```python
from build123d import *

# Parameters (mm, degrees)
F1_DEPTH      = 42
F2_T          = -3.5
F3_W          = 40
F3_H          = 75
F4_DEPTH      = 4
F6_DEPTH      = 5
F8_W          = 9
F8_H          = 9
F9_DEPTH      = 20.5
F10_DEPTH     = 32
F12_R         = 6
F13_DEPTH     = 25
F15_W         = 8.3580343053
F15_H         = 30.4632759653
F15_W_2       = 12.1421813965
F15_H_2       = 30.5070821196
F16_DEPTH     = 6
F17_T1_DEPTH  = 169.3882617949
F17_T3_DEPTH  = 92.6602540378
F17_T5_DEPTH  = 46.118363099
F17_T7_DEPTH  = 35
F18_D         = 2.5
F18_DEPTH     = 18
F18_TIP       = 0.7510757738
F19_T1_DEPTH  = 80
F19_T6_DEPTH  = 2
F19_T12_DEPTH = 2
F20_D         = 2.5
F20_DEPTH     = 18
F20_TIP       = 0.7510757738


# Not quite as in the source:
# - a fillet or chamfer that OpenCascade refuses, or shapes differently, is made with other operations: its cross-section is extruded or revolved along the edge and cut away or added
# - a feature names something its author has since deleted; it is built from what else it names


with BuildPart() as f1:
    # F0 (on Front) → F1 (new body, symmetric)
    with BuildSketch(Plane.XZ):
        Polygon((-66.6393345791, 36.118363099), (-66.6393345791, 0), (93.3606654209, 0), (93.3606654209, 25), (-65.6393345791, 36.118363099), align=None)
    extrude(amount=F1_DEPTH, both=True)

    # F2
    f2_openings = [f1.faces().sort_by_distance(p)[0] for p in [
        (13.360665, 0, 0),
    ]]
    offset(amount=F2_T, openings=f2_openings)

    # F3 (on face) → F4 (cut)
    with BuildSketch(Plane(origin=(2.1939535511, 0, 31.3749975164), x_dir=(0.9975640503, 0, -0.0697564737), z_dir=(0.0697564737, 0, 0.9975640503))):
        with Locations((-20.9989301063, 0)):
            Rectangle(F3_W, F3_H)
    extrude(amount=-F4_DEPTH, mode=Mode.SUBTRACT)

    # F3 (on face) → F6 (cut)
    with BuildSketch(Plane(origin=(2.1939535511, 0, 31.3749975164), x_dir=(0.9975640503, 0, -0.0697564737), z_dir=(0.0697564737, 0, 0.9975640503))):
        with BuildLine():
            Line((14.9393316886, 27.279802623), (14.9393316886, 22.720197377))
            ThreePointArc((14.9393316886, 22.720197377), (19.3893316886, 20), (23.8393316886, 22.720197377))
            Line((23.8393316886, 22.720197377), (23.8393316886, 27.279802623))
            ThreePointArc((23.8393316886, 27.279802623), (19.3893316886, 30), (14.9393316886, 27.279802623))
        make_face()
        with BuildLine():
            Line((20.0393316886, -34.0238362551), (20.0393316886, -33.0238362551))
            ThreePointArc((20.0393316886, -33.0238362551), (19.3893316886, -16.9498789917), (18.7393316886, -33.0238362551))
            Line((18.7393316886, -33.0238362551), (18.7393316886, -34.0238362551))
            Line((18.7393316886, -34.0238362551), (20.0393316886, -34.0238362551))
        make_face()
    extrude(amount=-F6_DEPTH, mode=Mode.SUBTRACT)

    # F8 (on offset) → F9 (join)
    with BuildSketch(Plane(origin=(0, 0, 2.5), x_dir=(1, 0, 0), z_dir=(0, 0, -1))):
        with Locations((81.6606654209, 34)):
            Rectangle(F8_W, F8_H)
        with Locations((81.6606654209, -34)):
            Rectangle(F8_W, F8_H)
    extrude(amount=-F9_DEPTH)

    # F8 (on offset) → F10 (join)
    with BuildSketch(Plane(origin=(0, 0, 2.5), x_dir=(1, 0, 0), z_dir=(0, 0, -1))):
        with Locations((-58.6393345791, -34)):
            Rectangle(F8_W, F8_H)
        with Locations((-58.6393345791, 34)):
            Rectangle(F8_W, F8_H)
    extrude(amount=-F10_DEPTH)

    # F12 (on offset) → F13 (cut)
    with BuildSketch(Plane(origin=(-66.6393345791, 0, 0), x_dir=(0, -1, 0), z_dir=(-1, 0, 0))):
        with Locations((-22, 23)):
            Circle(F12_R)
        with Locations((22, 23)):
            Circle(F12_R)
    extrude(amount=-F13_DEPTH, mode=Mode.SUBTRACT)

    # F15 (on offset) → F16 (join)
    with BuildSketch(Plane(origin=(1.949805893, 0, 27.8835233405), x_dir=(0.9975640503, 0, -0.0697564737), z_dir=(-0.0697564737, 0, -0.9975640503))):
        with Locations((5.292899441, 1.1196539272)):
            Rectangle(F15_W, F15_H)
        with Locations((44.2803874612, 1.1346279643)):
            Rectangle(F15_W_2, F15_H_2)
    extrude(amount=F16_DEPTH)

    # F17: fillet of radius 2 on 7 edges, made by hand

    # F17_s2 → F17_t1 (cut)
    with BuildSketch(Plane(origin=(96.1545321211, 0, -6.7237798852), x_dir=(0, 1, 0), z_dir=(-0.9975640503, 0, 0.0697564737))):
        with BuildLine():
            ThreePointArc((40, -31.4516120627), (41.4142135624, -30.865825625), (42, -29.4516120627))
            Line((42, -29.4516120627), (42, -31.4516120627))
            Line((42, -31.4516120627), (40, -31.4516120627))
        make_face()
        with BuildLine():
            ThreePointArc((-40, -31.4516120627), (-41.4142135624, -30.865825625), (-42, -29.4516120627))
            Line((-42, -29.4516120627), (-42, -31.4516120627))
            Line((-42, -31.4516120627), (-40, -31.4516120627))
        make_face()
    extrude(amount=F17_T1_DEPTH, mode=Mode.SUBTRACT)

    # F17_s4 → F17_t3 (cut)
    with BuildSketch(Plane.XZ.offset(-46.3301270189)):
        with BuildLine():
            ThreePointArc((-65.6393345791, 36.118363099), (-66.3713853867, 35.3863122914), (-66.6393345791, 34.3863122914))
            Line((-66.6393345791, 34.3863122914), (-66.6393345791, 36.118363099))
            Line((-66.6393345791, 36.118363099), (-65.6393345791, 36.118363099))
        make_face()
    extrude(amount=F17_T3_DEPTH, mode=Mode.SUBTRACT)

    # F17_s6 → F17_t5 (cut)
    with BuildSketch(Plane.XY.offset(-5)):
        with BuildLine():
            ThreePointArc((-64.6393345791, 42), (-66.0535481415, 41.4142135624), (-66.6393345791, 40))
            Line((-66.6393345791, 40), (-66.6393345791, 42))
            Line((-66.6393345791, 42), (-64.6393345791, 42))
        make_face()
        with BuildLine():
            ThreePointArc((-64.6393345791, -42), (-66.0535481415, -41.4142135624), (-66.6393345791, -40))
            Line((-66.6393345791, -40), (-66.6393345791, -42))
            Line((-66.6393345791, -42), (-64.6393345791, -42))
        make_face()
    extrude(amount=F17_T5_DEPTH, mode=Mode.SUBTRACT)

    # F17_s8 → F17_t7 (cut)
    with BuildSketch(Plane.XY.offset(-5)):
        with BuildLine():
            ThreePointArc((91.3606654209, 42), (92.7748789833, 41.4142135624), (93.3606654209, 40))
            Line((93.3606654209, 40), (93.3606654209, 42))
            Line((93.3606654209, 42), (91.3606654209, 42))
        make_face()
        with BuildLine():
            ThreePointArc((93.3606654209, -40), (92.7748789833, -41.4142135624), (91.3606654209, -42))
            Line((91.3606654209, -42), (93.3606654209, -42))
            Line((93.3606654209, -42), (93.3606654209, -40))
        make_face()
    extrude(amount=F17_T7_DEPTH, mode=Mode.SUBTRACT)

    # F18
    with Locations(Plane(origin=(0, 0, 2.5), x_dir=(1, 0, 0), z_dir=(0, 0, -1))):
        with Locations((-58.6393345791, 34), (-58.6393345791, -34)):
            Hole(F18_D / 2, depth=F18_DEPTH)
            with Locations((0, 0, -(F18_DEPTH + F18_TIP / 2))):  # 118° drill point
                Cone(0, F18_D / 2, F18_TIP, mode=Mode.SUBTRACT)

    # F19: fillet of radius 2 on 1 edges, made by hand

    # F19_s2 → F19_t1 (cut)
    with BuildSketch(Plane.XZ.offset(-40)):
        with BuildLine():
            ThreePointArc((91.5001783684, 25.1300979282), (92.8233728241, 24.4989665478), (93.3606654209, 23.1349698277))
            Line((93.3606654209, 23.1349698277), (93.3606654209, 25))
            Line((93.3606654209, 25), (91.5001783684, 25.1300979282))
        make_face()
    extrude(amount=F19_T1_DEPTH, mode=Mode.SUBTRACT)


with BuildPart() as f19_tool4:
    # F19_s5 → F19_t6 (new body)
    with BuildSketch(Plane.XZ.offset(40)):
        Polygon((91.3606654209, 23.1349698277), (91.5001783684, 25.1300979282), (93.3606654209, 25), (93.3606654209, 23.1349698277), align=None)
    extrude(amount=F19_T6_DEPTH)

    # F19_s7 → F19_t8 (revolve, cut)
    with BuildSketch(Plane(origin=(91.3606654209, -40, 23.1349698277), x_dir=(-0.7313537016, 0, -0.6819983601), z_dir=(-0.6819983601, 0, 0.7313537016))):
        with BuildLine():
            ThreePointArc((0, -2), (2, 0), (0, 2))
            Line((0, 2), (0, -2))
        make_face()
    revolve(axis=Axis((91.3606654209, -40, 23.1349698277), (0, -1, 0)), mode=Mode.SUBTRACT)


with BuildPart() as f1_1:
    add(f1.part)

    # F19_t3: cut F19_tool4
    add(f19_tool4.part, mode=Mode.SUBTRACT)


with BuildPart() as f19_tool10:
    # F19_s11 → F19_t12 (new body)
    with BuildSketch(Plane.XZ.offset(-40)):
        Polygon((91.3606654209, 23.1349698277), (91.5001783684, 25.1300979282), (93.3606654209, 25), (93.3606654209, 23.1349698277), align=None)
    extrude(amount=-F19_T12_DEPTH)

    # F19_s13 → F19_t14 (revolve, cut)
    with BuildSketch(Plane(origin=(91.3606654209, 40, 23.1349698277), x_dir=(-0.7313537016, 0, -0.6819983601), z_dir=(0.6819983601, 0, -0.7313537016))):
        with BuildLine():
            ThreePointArc((0, -2), (2, 0), (0, 2))
            Line((0, 2), (0, -2))
        make_face()
    revolve(axis=Axis((91.3606654209, 40, 23.1349698277), (0, 1, 0)), mode=Mode.SUBTRACT)


with BuildPart() as f1_2:
    add(f1_1.part)

    # F19_t9: cut F19_tool10
    add(f19_tool10.part, mode=Mode.SUBTRACT)

    # F20
    with Locations(Plane(origin=(0, 0, 2.5), x_dir=(1, 0, 0), z_dir=(0, 0, -1))):
        with Locations((81.6606654209, 34), (81.6606654209, -34)):
            Hole(F20_D / 2, depth=F20_DEPTH)
            with Locations((0, 0, -(F20_DEPTH + F20_TIP / 2))):  # 118° drill point
                Cone(0, F20_D / 2, F20_TIP, mode=Mode.SUBTRACT)


solid = f1_2.part
```
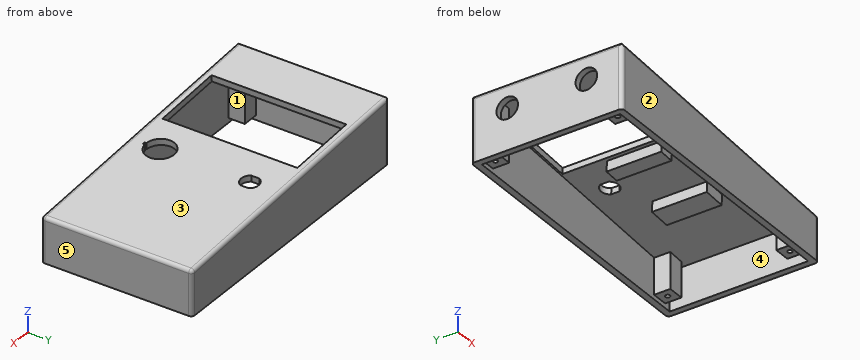
Geometry check sheet. Reference: the model listing, model coordinates, mm. Face numbers are marked on the shaded views. A direction names the side the tool comes from. Coordinates: 2 decimals unless noted, no trailing zeros. Loops run counter-clockwise (first coordinate to the right, second up) from the corner with the lowest first, then second, coordinate; pieces in that order, holes last. Notation, with made-up numbers: (-18.5, 71) - (12.5, 71) arc R32 cw to (12.5, 102) - close; hole circle Ø8 at (64.25, -8). An arc over 180 degrees is marked (long way). One line per item, written item: value. Start each with the question number.
(1) Cross-section at A-A on z = 13. Enter the section's corners in (x, y).
(2) Mould release check, pull along X, two halves, no side actions. Record for the marked faces 1, 2 and 3: released by +X, released by -X, zero draft, split by the parting line, or undercut.
(3) Cross-section at B-B on y = -18.5. Enter the section's corners in (x, z) (3 decimals).
(4) Depth check by flat-ended pin: P1, Ø2, axis at x = -58.64, y = -34, coming from the -Z side; P2, Ø4.5, axis at x = -56.5, y = 32, coming from the -Z side; P3, Ø1.5, axis at x = 54.5, y = 12.5, coming from the +Z side. Enter the tip coordinate at first touch or a pass-through.
(5) Cross-section at C-C on y = 24.5. Enter the section's corners in (x, z) (3 decimals).
(6) Tool access check on the marked faces 4 and 5. Record the directions out of +Z, -Z, +X, -X, +Y, -Y that give a thin tool (end or side, any length) a straight path to the whole face; none if there is none.
(7) Material ranges on line 1 (X direction, y = 34, z = 10.25); line 2 (Z direction, x = -65.4, y = 22); line 3 (Y direction, x = -50.5, z = 20), recorded low to high. Write a range as [from, to].
Results below:
1. outline: (-66.64, -40) arc R2 ccw to (-64.64, -42) - (91.36, -42) arc R2 ccw to (93.36, -40) - (93.36, 40) arc R2 ccw to (91.36, 42) - (-64.64, 42) arc R2 ccw to (-66.64, 40) - close; hole (-63.14, -29.5) - (-54.14, -29.5) - (-54.14, -38.5) - (77.16, -38.5) - (77.16, -29.5) - (86.16, -29.5) - (86.16, -38.5) - (89.86, -38.5) - (89.86, 38.5) - (86.16, 38.5) - (86.16, 29.5) - (77.16, 29.5) - (77.16, 38.5) - (-54.14, 38.5) - (-54.14, 29.5) - (-63.14, 29.5) - close; hole circle Ø2.5 at (-58.64, -34); hole circle Ø2.5 at (-58.64, 34); hole circle Ø2.5 at (81.66, -34); hole circle Ø2.5 at (81.66, 34)
2. face 1: undercut
2. face 2: zero draft
2. face 3: released by +X
3. outline: (-66.639, 0) - (-63.139, 0) - (-63.139, 18.127) - (-66.639, 18.127) - close; (-66.639, 27.873) - (-63.139, 27.873) - (-63.139, 32.435) - (-38.949, 30.743) - (-38.705, 34.235) - (-65.639, 36.118) arc R2 ccw to (-66.639, 34.386) - close; (0.953, 27.953) - (16.554, 26.862) - (16.798, 30.354) - (1.197, 31.445) - close; (26.029, 26.2) - (89.861, 21.736) - (89.861, 0) - (93.361, 0) - (93.361, 23.135) arc R2 ccw to (91.5, 25.13) - (26.274, 29.691) - close
4. P1: stops at z = 20.65
4. P2: stops at z = 2.5
4. P3: stops at z = 27.77
5. outline: (-66.639, 0) - (-63.139, 0) - (-63.139, 17.546) - (-66.639, 17.546) - close; (-66.639, 28.454) - (-63.139, 28.454) - (-63.139, 32.435) - (-38.949, 30.743) - (-38.705, 34.235) - (-65.639, 36.118) arc R2 ccw to (-66.639, 34.386) - close; (0.953, 27.953) - (16.853, 26.841) - (17.097, 30.333) - (1.197, 31.445) - close; (25.731, 26.221) - (89.861, 21.736) - (89.861, 0) - (93.361, 0) - (93.361, 23.135) arc R2 ccw to (91.5, 25.13) - (25.975, 29.712) - close
6. face 4: -Z
6. face 5: +Z, -Z, +X, +Y, -Y
7. line 1: x = [-66.64, -59.89], [-57.39, -54.14], [77.16, 80.41], [82.91, 86.16], [89.86, 93.36]
7. line 2: z = [0, 17], [29, 36.1]
7. line 3: y = [-42, -38.5], [38.5, 42]
